Geometry: see drawing. Coordinates: mm, zero at the bounding-box minimum. A direction names the side the tool comes from. Round coordinates to 2 decimals unless told otherwise and drop trailing zeros. Write each loop counter-clockwise with the first axis right and the second up, starting at its lowest first coordinate (ties: lowest second). Pieces come first, ordered by that corner, then holes. Notation, with made-up numbers: (26, 42.25) -> (55, 42.25) arc R21 ccw to (55, 47.25) -> close; hole circle Ø6 at (-1.5, 74.5). An arc over 180 degrees is marked (long way). Write item = value, one per line. Start each with the question number.
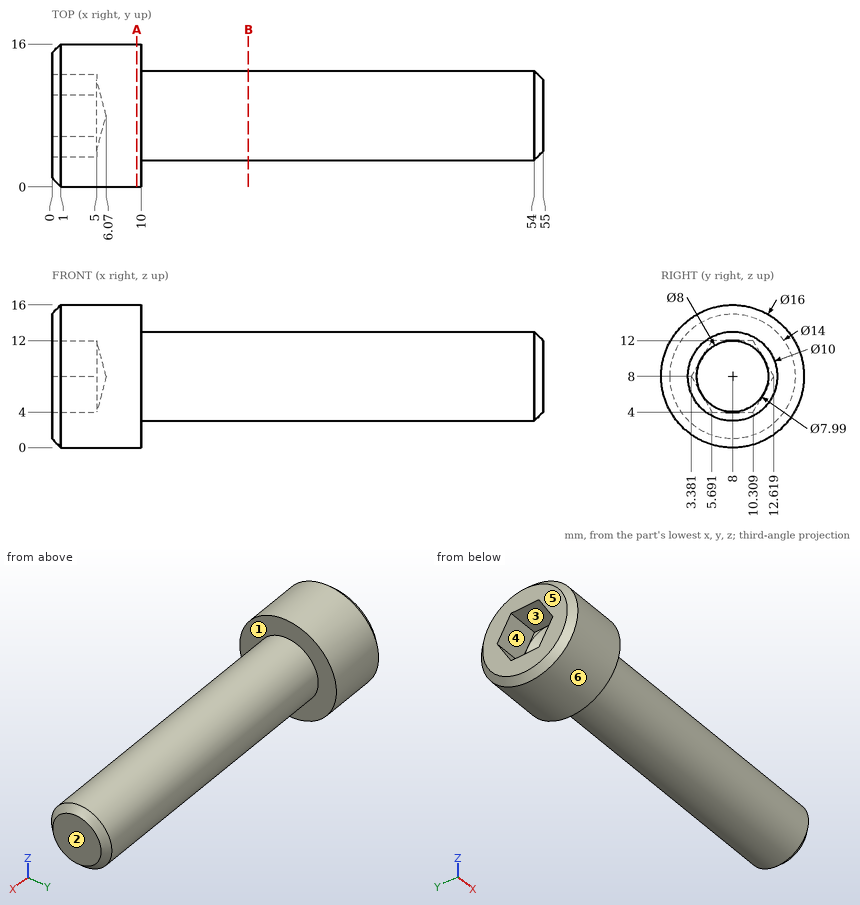
1. Section A-A (x = 9.5). Output: boundary loops of the cut face in (y, z), then the cut area to 3 significant figures.
2. Section B-B (x = 22). Output: boundary loops of the cut face in (y, z).
3. Pin query (flat end, axial travel): P1, Ø3, axis at x = 48.5, y = 7.5, coming from the +Z side; P2, Ø4, axis at x = 33.5, z = 10.5, coming from the +Y side (1 decimal); P3, Ø6, axis at x = 48, z = 14, coming from the -Y side. Return the tip coordinate at first contact, or that it passes through.
4. Mould query, pull axis Z, two halves, no side actions, for the marked faces 4, 5 and 6. Classes: pulls with the +Z half, pulls with the -Z half, needs draft (parallel to the pull), parting line crosses it, or undercut.
5. Line query: line 1 along X through (y, z) = (3.75, 12.75); line 2 along Z through (x, y) = (4, 6) (1 decimal); line 3 along Y through (x, z) = (49, 6.25) (1 decimal). Output: solid intervals per line, ascending.
6. Reachability of the marked faces 1, 2 and 3 from +Z, -Z, +X, -X, +Y, -Y: full face, straight path, thin tool, end or side. Return the list, or none.
Check sheet entries:
q1.outline = circle Ø16 at (8, 8)
q1.area = 201 mm2
q2.outline = circle Ø10 at (8, 8)
q3.P1 = 13
q3.P2 = 13
q3.P3 = 4
q4.face_4 = undercut
q4.face_5 = needs draft
q4.face_6 = parting line crosses it
q5.line_1 = 0 to 10
q5.line_2 = 0.3 to 4, 12 to 15.7
q5.line_3 = 3.3 to 12.7
q6.face_1 = +X
q6.face_2 = +Z, -Z, +X, +Y, -Y
q6.face_3 = -X
